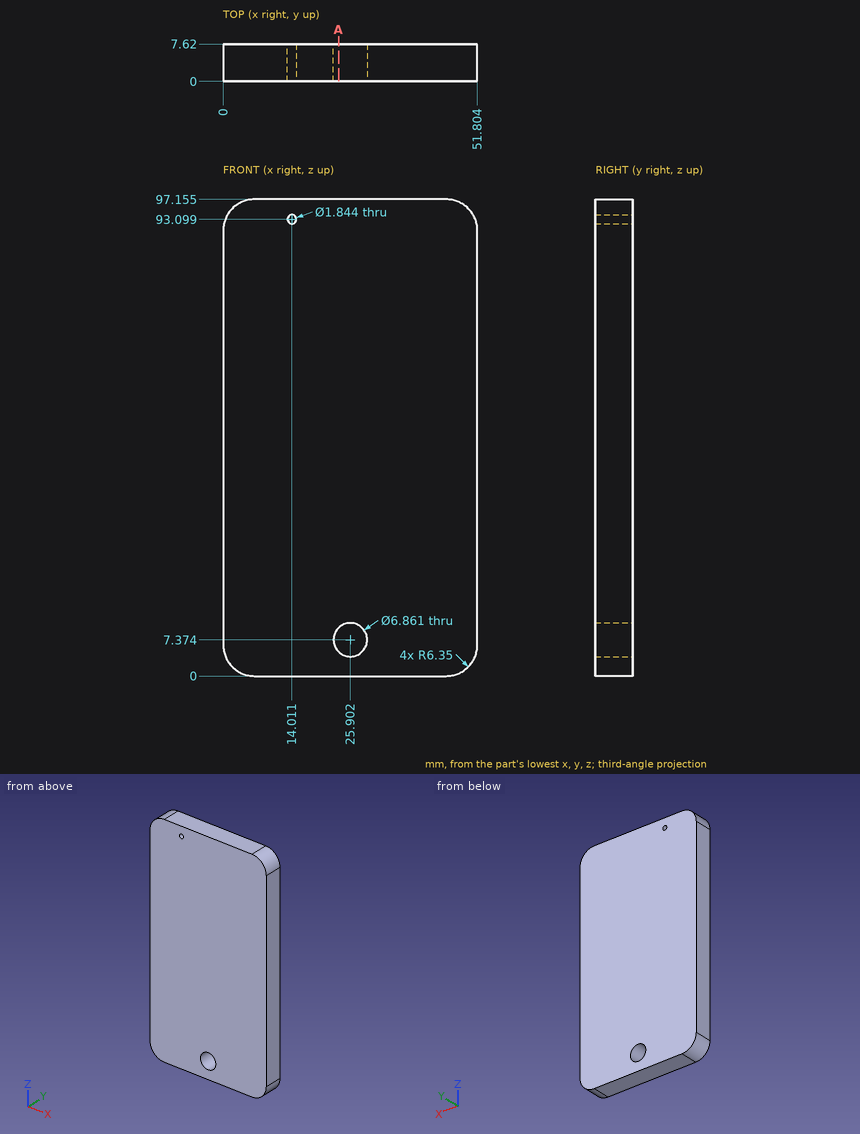
Part print with two shaded views. Sizes in mm from the minimum x, y, z corner. Give positions to 0.01 mm unless a question says otherwise; leave off trailing zeros. Order: outer loops, then holes, each group sorted by start corner. A loop starts at its lowest first (then second) coordinate and runs counter-clockwise, first axis right, second up. Notation, with made-up numbers: M 60.25,23 L 107.25,23 A28 ccw 107.25,58 Z; hole C -35,41 d5. An arc over 180 degrees is marked long. Put each result on its own line as item: value.
Item 1: Drop a flat-ended pin along its axis: pin 1 Ø1.1 at (x, z) = (14.01, 93.1) entering from +Y. Give the stop position or say it passes through.
Results are:
pin 1: through
Item 2: Cut at A-A on x = 23.5. Write the cut outline in (y, z) (1 decimal), then the cut area to 3 significant figures.
Results are:
outline: M 0,0 L 7.6,0 L 7.6,4.9 L 0,4.9 Z; M 0,9.8 L 7.6,9.8 L 7.6,97.2 L 0,97.2 Z
area: 703 mm2
Item 3: Wall check: probe 1 along Z at (x, y) = (26, 5.5) (1 decimal); probe 2 along X at (y, z) = (7.25, 5.5) (1 decimal); probe 3 along Z at (x, y) = (28, 7) (1 decimal). Give the ranges that are in metal, low to high.
Results are:
probe 1: 0 to 3.9, 10.8 to 97.2
probe 2: 0.1 to 23, 28.8 to 51.7
probe 3: 0 to 4.7, 10.1 to 97.2
